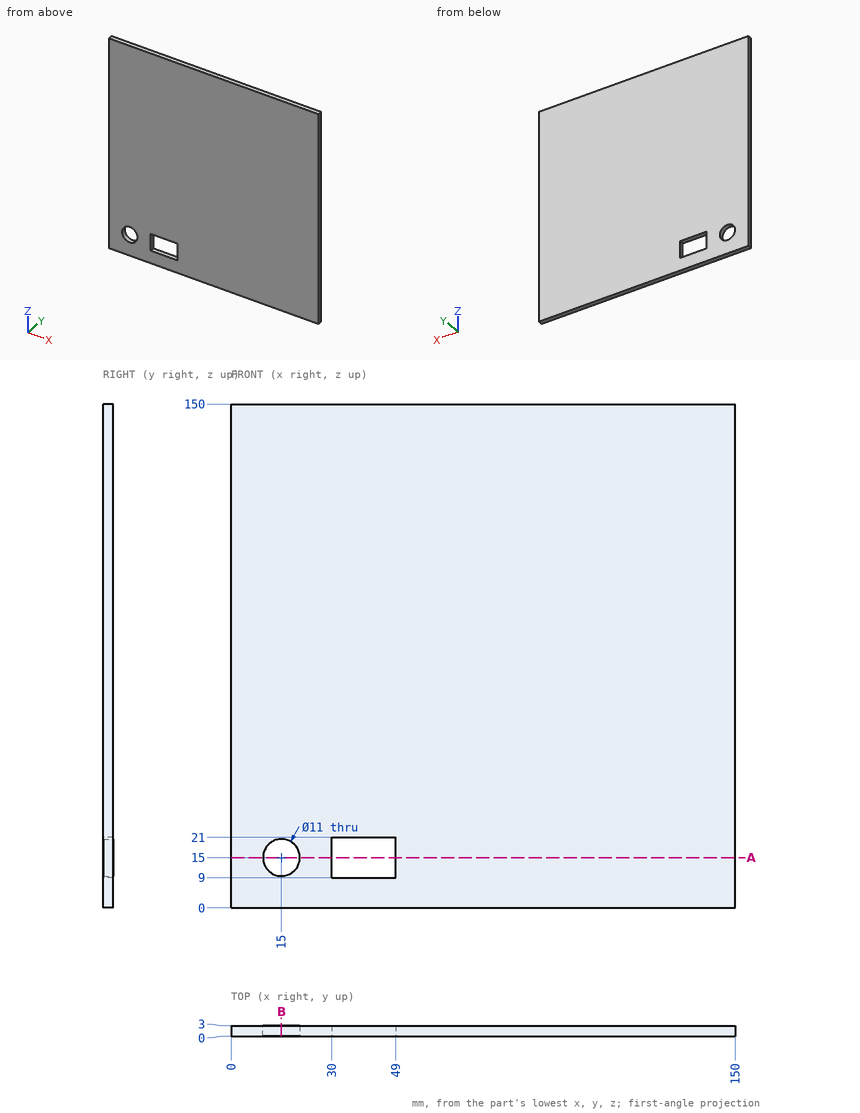
For this review, use the dimensioned drawing (mm, ordinates from the lowest corner) and the shaded views. Give positions to 0.01 mm unless a question says otherwise; leave off trailing zeros. Order: outer loops, then holes, each group sorted by start corner. A loop starts at its lowest first (then second) coordinate and runs counter-clockwise, first axis right, second up. Notation, with made-up numbers: (-19.75, 28) - (38.25, 28) arc R18 ccw to (38.25, 42) - close; hole circle Ø7 at (-20, 0.25). An arc over 180 degrees is marked (long way). Use CSV: the item, a comma, the result in double quotes. Start each with the question number.
Q1. Clearance check with flat-ended pins moving along their axes: pin 1 Ø0.9 at (y, z) = (2, 15) entering from -X; pin 2 Ø10 at (x, z) = (15, 15) entering from -Y. State where each tip first meets the part, or that it passes through.
Q2. We need section B-B, the plane x = 15. Write out the cut boundary in (y, z).
Q3. We need section A-A, the plane z = 15. Write out the cut boundary in (x, y).
Q4. To check wall thickness, follow line 1 along Z through (x, y) = (15, 1.9); line 2 along Z through (x, y) = (33, 1.9); line 3 along X through (y, z) = (2.2, 11). State the ranges of each line that lie inside material, in increasing order. Write a range as [from, to].
Outcome:
1,pin 1,"stops at x = 0"
1,pin 2,"passes through"
2,outline,"(0, 0) - (3, 0) - (3, 9.5) - (0, 9.5) - close; (0, 20.5) - (3, 20.5) - (3, 150) - (0, 150) - close"
3,outline,"(0, 0) - (9.5, 0) - (9.5, 3) - (0, 3) - close; (20.5, 0) - (30, 0) - (30, 3) - (20.5, 3) - close; (49, 0) - (150, 0) - (150, 3) - (49, 3) - close"
4,line 1,"z = [0, 9.5], [20.5, 150]"
4,line 2,"z = [0, 9], [21, 150]"
4,line 3,"x = [0, 11.23], [18.77, 30], [49, 150]"
